Read the model definition and answer for the solid it produces. Units are mm, in the model's axes. Give positions to 0.01 mm unless a question says otherwise; leave off trailing zeros. Order: outer loops, then holes, each group sorted by start corner. A loop starts at its lowest first (then second) coordinate and runs counter-clockwise, first axis right, second up. Notation, with made-up numbers: (48, 43.25) - (85, 43.25) arc R14 cw to (85, 58.25) - close; hole circle Ø8 at (7.5, -3.5). An arc over 180 degrees is marked (long way). One line per item, written item: value. Start each with the question number.
```python
from build123d import *

# Parameters (mm, degrees)
ESBO_O1_W                = 7.2
ESBO_O1_H                = 14
ESBO_O1_R                = 1.5
RESSALTO_EXTRUS_O1_DEPTH = 3
FILETE1_R                = 2


with BuildPart() as part:
    # Esboço1 → Ressalto-extrusão1 (new body)
    with BuildSketch(Plane.XY):
        with Locations((3.6, 7)):
            Rectangle(ESBO_O1_W, ESBO_O1_H)
        with Locations((3.6, 8.5)):
            Circle(ESBO_O1_R, mode=Mode.SUBTRACT)
    extrude(amount=RESSALTO_EXTRUS_O1_DEPTH)

    # Filete1
    filete1_edges = [part.edges().sort_by_distance(p)[0] for p in [
        (0, 14, 1.5),
        (7.2, 14, 1.5),
    ]]
    fillet(filete1_edges, radius=FILETE1_R)


solid = part.part
```
1) Section D-D on x = 6.5 is taken. Write down the section's boundary in (y, z), plus the area to 3 significant figures.
2) Find the intervals of material crossed by probe 1 along Y at (x, z) = (3.6, 2.3); probe 2 along Y at (x, z) = (4.5, 2.7); probe 3 along X at (y, z) = (9.5, 0.9), in increasing order. Write a range as from..to.
3) Section C-C on z = 1.15 is taken. Write down the section's boundary in (x, y).
4) Section A-A on y = 8.5 is taken. Write down the section's boundary in (x, z).
5) The mould has two halves that part along Y. Classify faces 1 (the cylindrical face through (4.29, 7.17, 1.48)), 2 (the flat face through (4, 0, 1)), 3 (the flat face through (2.7, 7.1, 0)), 4 (the flat face through (4, 14, 1)): +Y half, -Y half, draft (parallel to the pull), parting line (faces both ways), or undercut.
6) Section B-B on x = 3.6 is taken. Write down the section's boundary in (y, z).
Solved:
1. outline: (0, 0) - (13.52, 0) - (13.52, 3) - (0, 3) - close
1. area: 40.6 mm2
2. probe 1: y = 0..7, 10..14
2. probe 2: y = 0..7.3, 9.7..14
2. probe 3: x = 0..2.48, 4.72..7.2
3. outline: (0, 0) - (7.2, 0) - (7.2, 12) arc R2 ccw to (5.2, 14) - (2, 14) arc R2 ccw to (0, 12) - close; hole circle Ø3 at (3.6, 8.5)
4. outline: (0, 0) - (2.1, 0) - (2.1, 3) - (0, 3) - close; (5.1, 0) - (7.2, 0) - (7.2, 3) - (5.1, 3) - close
5. face 1: undercut
5. face 2: -Y half
5. face 3: draft
5. face 4: +Y half
6. outline: (0, 0) - (7, 0) - (7, 3) - (0, 3) - close; (10, 0) - (14, 0) - (14, 3) - (10, 3) - close
